from build123d import *

# Parameters (mm, degrees)
SKETCH021_W  = 22
SKETCH021_H  = 12.704962
PAD014_DEPTH = 10
SKETCH020_R  = 2.5
PAD013_DEPTH = 2
SKETCH015_R  = 1.5
PAD008_DEPTH = 60
SKETCH019_R  = 1.6
PAD012_DEPTH = 5
PAD005_DEPTH = 2
SKETCH018_W  = 11
SKETCH018_H  = 5.369358
PAD011_DEPTH = 26.5
SKETCH022_W  = 21.583895
SKETCH022_H  = 15.194446
PAD015_DEPTH = 60
SKETCH010_R  = 6
PAD003_DEPTH = 3
SKETCH009_W  = 30
SKETCH009_H  = 9
PAD002_DEPTH = 80.5
SKETCH008_R  = 1.4
PAD001_DEPTH = 14
SKETCH013_W  = 3.5
SKETCH013_H  = 26
PAD006_DEPTH = 3
SKETCH_W     = 44
SKETCH_H     = 64
PAD_DEPTH    = 14
PAD007_DEPTH = 12
CHAMFER_SIZE = 3


with BuildPart() as pad014:
    # Sketch021 → Pad014 (new body)
    with BuildSketch(Plane.XZ.offset(-81)):
        with Locations((41, 11.352481)):
            Rectangle(SKETCH021_W, SKETCH021_H)
    extrude(amount=PAD014_DEPTH)


with BuildPart() as obj1:
    # Sketch020 → Pad013 (new body)
    with BuildSketch(Plane.XY):
        with Locations((10, -0.5)):
            Circle(SKETCH020_R)
        with Locations((19.5, -0.5)):
            Circle(SKETCH020_R)
    extrude(amount=PAD013_DEPTH)


with BuildPart() as obj2:
    # Sketch015 → Pad008 (new body)
    with BuildSketch(Plane.YZ):
        with Locations((40.5, 12)):
            Circle(SKETCH015_R)
        with BuildLine():
            ThreePointArc((53.5, 13.5), (52, 12), (53.5, 10.5))
            Line((53.5, 10.5), (56.5, 10.5))
            ThreePointArc((56.5, 10.5), (58, 12), (56.5, 13.5))
            Line((53.5, 13.5), (56.5, 13.5))
        make_face()
    extrude(amount=PAD008_DEPTH)


with BuildPart() as endstopmount:
    # Sketch019 → Pad012 (new body)
    with BuildSketch(Plane.XY):
        with Locations((10, -0.5)):
            Circle(SKETCH019_R)
        with Locations((19.5, -0.5)):
            Circle(SKETCH019_R)
    extrude(amount=PAD012_DEPTH)


with BuildPart() as obj3:
    # Sketch006 → Pad005 (new body)
    with BuildSketch(Plane(origin=(0, -9.25, 3), x_dir=(1, 0, 0), z_dir=(0, 0, 1))):
        Polygon((5.55, 86.434679), (2.45, 86.434679), (0.9, 83.75), (2.45, 81.065321), (5.55, 81.065321), (7.1, 83.75), align=None)
        Polygon((57.55, 81.065321), (59.1, 83.75), (57.55, 86.434679), (54.45, 86.434679), (52.9, 83.75), (54.45, 81.065321), align=None)
        Polygon((0.9, 17.25), (2.45, 14.565321), (5.55, 14.565321), (7.1, 17.25), (5.55, 19.934679), (2.45, 19.934679), align=None)
        Polygon((52.9, 17.25), (54.45, 14.565321), (57.55, 14.565321), (59.1, 17.25), (57.55, 19.934679), (54.45, 19.934679), align=None)
    extrude(amount=PAD005_DEPTH)


with BuildPart() as obj4:
    # Sketch018 → Pad011 (new body, symmetric)
    with BuildSketch(Plane.YZ.offset(30)):
        Polygon((42.05, 9.315321), (43.6, 12), (42.05, 14.684679), (38.95, 14.684679), (37.4, 12), (38.95, 9.315321), align=None)
        with Locations((54.55, 12)):
            Rectangle(SKETCH018_W, SKETCH018_H)
    extrude(amount=PAD011_DEPTH, both=True)


with BuildPart() as cutblock02:
    # Sketch022 → Pad015 (new body)
    with BuildSketch(Plane.YZ):
        with Locations((-10.791947, 12.597223)):
            Rectangle(SKETCH022_W, SKETCH022_H)
    extrude(amount=PAD015_DEPTH)

    # Fusion002: union Pad014, obj1, obj2, EndstopMount, obj3, obj4
    add(pad014.part)
    add(obj1.part)
    add(obj2.part)
    add(endstopmount.part)
    add(obj3.part)
    add(obj4.part)


with BuildPart() as springhole:
    # Sketch010 → Pad003 (new body)
    with BuildSketch(Plane.XZ.offset(-7)):
        with Locations((40.5, 7)):
            Circle(SKETCH010_R)
    extrude(amount=PAD003_DEPTH)


with BuildPart() as profile:
    # Sketch009 → Pad002 (new body)
    with BuildSketch(Plane.XZ):
        with Locations((15, 9.5)):
            Rectangle(SKETCH009_W, SKETCH009_H)
        Polygon((52, 5), (45, 14), (60, 14), (60, 5), align=None)
    extrude(amount=-PAD002_DEPTH)


with BuildPart() as mounthole:
    # Sketch008 → Pad001 (new body)
    with BuildSketch(Plane.XY):
        with Locations((4, 8)):
            Circle(SKETCH008_R)
        with Locations((56, 8)):
            Circle(SKETCH008_R)
        with Locations((4, 74.5)):
            Circle(SKETCH008_R)
        with Locations((56, 74.5)):
            Circle(SKETCH008_R)
    extrude(amount=PAD001_DEPTH)


with BuildPart() as cutblocks:
    # Sketch013 → Pad006 (new body)
    with BuildSketch(Plane.XY.offset(5)):
        with Locations((6.25, 47.5)):
            Rectangle(SKETCH013_W, SKETCH013_H)
        with Locations((53.75, 47.5)):
            Rectangle(SKETCH013_W, SKETCH013_H)
    extrude(amount=-PAD006_DEPTH)

    # Fusion001: union SpringHole, Profile, MountHole
    add(springhole.part)
    add(profile.part)
    add(mounthole.part)


with BuildPart() as cut:
    # Sketch → Pad (new body)
    with BuildSketch(Plane.XY):
        Polygon((60, 80.5), (60, 0), (52.5, -7.5), (7.5, -7.5), (0, 0), (0, 80.5), align=None)
        with Locations((30, 39)):
            Rectangle(SKETCH_W, SKETCH_H, mode=Mode.SUBTRACT)
    extrude(amount=PAD_DEPTH)

    # Cut: cut CutBlocks
    add(cutblocks.part, mode=Mode.SUBTRACT)


with BuildPart() as chamfer_body:
    # Sketch014 → Pad007 (new body)
    with BuildSketch(Plane.XY.offset(5)):
        Polygon((4.5, 60.5), (4.5, 34.5), (8, 34.5), (8, 31.5), (0, 31.5), (0, 63.5), (8, 63.5), (8, 60.5), align=None)
        Polygon((55.5, 60.5), (55.5, 34.5), (52, 34.5), (52, 31.5), (60, 31.5), (60, 63.5), (52, 63.5), (52, 60.5), align=None)
    extrude(amount=PAD007_DEPTH)

    # Fusion: union Cut
    add(cut.part)

    # Cut001: cut CutBlock02
    add(cutblock02.part, mode=Mode.SUBTRACT)

    # Chamfer
    chamfer_edges = [chamfer_body.edges().sort_by_distance(p)[0] for p in [
        (0, 80.5, 2.5),
        (0, 63.5, 11),
        (60, 63.5, 11),
        (60, 80.5, 2.5),
        (0, 31.5, 11),
        (60, 31.5, 11),
    ]]
    chamfer(chamfer_edges, length=CHAMFER_SIZE)


solid = chamfer_body.part
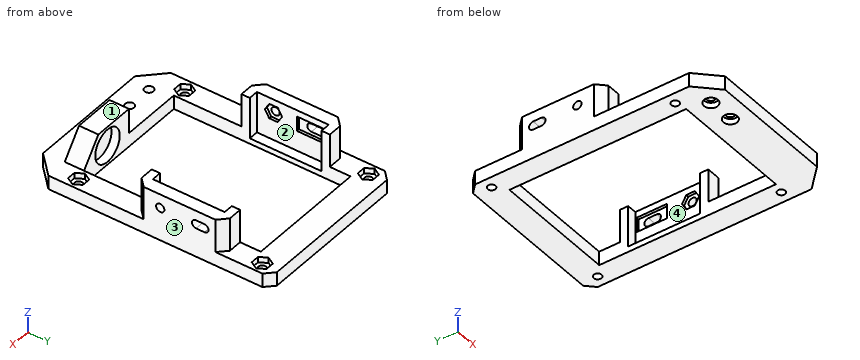
Can you work these out from the model? Positions are in its coordinate system, mm. Face numbers are marked on the shaded views. A direction names the side the tool comes from. Coordinates: 2 decimals unless noted, no trailing zeros. Loops run counter-clockwise (first coordinate to the right, second up) from the corner with the lowest first, then second, coordinate; pieces in that order, holes last. Notation, with made-up numbers: M 76,60 L 116,60 A27 cw 116,90 Z; hole C 33,84 d11. An arc over 180 degrees is marked long. Answer as CSV lines item,"result". Start each with the question number.
1. Suppose I cut it at C-C, the plane x = 10. List the corners of the cut face in (y, z) for me.
2. Suppose I cut it at B-B, the plane y = 40.5. List the corners of the cut face in (x, z) for me.
3. Suppose I cut it at D-D, the plane y = 27.5. List the corners of the cut face in (x, z) for me.
4. If I drill on probe 1 along Y at (x, z) = (10, 3.2); probe 2 along Y at (x, z) = (10, 0.55); probe 3 along X at (y, z) = (39.5, 6), over which ranges is the centre line in solid material (lowest first)? Write a range as [from, to].
5. Thinking about a two-plate mould opening in Y: for the marked faces 3 and 4, which applies, +Y half, -Y half, draft (parallel to the pull), parting line (faces both ways), or undercut?
6. For the marked faces 1 and 2, which set-ups out of +Z, -Z, +X, -X, +Y, -Y let a thin tool reach every point of the face, with its end or its side?
7. For pin 1 Ø2.5 at (y, z) = (40.5, 13) entering from +X; pin 2 Ø4 at (x, z) = (53, 7.5) entering from -Y; pin 3 Ø10 at (x, z) = (51.5, 14.5) entering from +Y; pin 4 Ø10 at (y, z) = (27, 10.5) entering from +X, each with a flat end and sliding along its axis, tell me the tip position at first contact or that it passes through.
8. Suppose I cut it at A-A, the plane x = 25.5. List the corners of the cut face in (y, z) for me.
Output:
1,outline,"M -7.5,0 L -3,0 L -3,2 L -2.1,2 L -2.1,5 L -7.5,5 Z; M 1.1,2 L 2,2 L 2,0 L 7,0 L 7,5 L 1.1,5 Z; M 71,0 L 80.5,0 L 80.5,5 L 71,5 Z"
2,outline,"M 0,0 L 8,0 L 8,2 L 4.5,2 L 4.5,9.32 L 3.5,9.32 L 3.5,10.5 L 0,10.5 Z; M 0,13.5 L 3.5,13.5 L 3.5,14.68 L 4.5,14.68 L 4.5,17 L 0,17 Z; M 52,0 L 60,0 L 60,10.5 L 56.5,10.5 L 56.5,9.32 L 55.5,9.32 L 55.5,2 L 52,2 Z; M 55.5,14.68 L 56.5,14.68 L 56.5,13.5 L 60,13.5 L 60,17 L 55.5,17 Z"
3,outline,"M 0,0 L 8,0 L 8,5 L 0,5 Z; M 52,0 L 60,0 L 60,5 L 52,5 Z"
4,probe 1,"y = [-7.5, -2.1], [1.1, 7], [71, 80.5]"
4,probe 2,"y = [-7.5, -3], [2, 7], [71, 80.5]"
4,probe 3,"x = [0, 4.5], [55.5, 60]"
5,face 3,"draft"
5,face 4,"undercut"
6,face 1,"+Z, +X, -X, +Y, -Y"
6,face 2,"+Z"
7,pin 1,"stops at x = 60"
7,pin 2,"stops at y = 31.5"
7,pin 3,"stops at y = 63.5"
7,pin 4,"stops at x = 57.5"
8,outline,"M -7.5,0 L 7,0 L 7,5 L -7.5,5 Z; M 71,0 L 80.5,0 L 80.5,5 L 71,5 Z"
